Here's how the part is built. I have some questions about the finished solid (model axes, mm). A direction names the side the tool comes from. Give positions to 0.01 mm unless a question says otherwise; leave off trailing zeros. Loops run counter-clockwise (first coordinate to the right, second up) from the corner with the lowest first, then second, coordinate; pieces in that order, holes last. Notation, with made-up numbers: (58, 3) - (86, 3) arc R26 ccw to (86, 41) - close; hole circle Ø1 at (58, -14). An arc over 180 degrees is marked (long way). Use one line per item in the form item = value.
from build123d import *

# Parameters (mm, degrees)
SKETCH1_R           = 10
SKETCH1_R_2         = 5
BOSS_EXTRUDE1_DEPTH = 30
FILLET1_R           = 3


with BuildPart() as part:
    # Sketch1 → Boss-Extrude1 (new body)
    with BuildSketch(Plane.XY):
        Circle(SKETCH1_R)
        Circle(SKETCH1_R_2, mode=Mode.SUBTRACT)
    extrude(amount=BOSS_EXTRUDE1_DEPTH)

    # Sketch4 → Revolve1 (revolve)
    with BuildSketch(Plane(origin=(0, 0, 0), x_dir=(1, 0, 0), z_dir=(0, 1, 0))):
        Polygon((10, -5), (30, -5), (30, -7), (25, -9.886751346), (25, -20.113248654), (30, -23), (30, -25), (10, -25), align=None)
    revolve(axis=Axis((0, 0, 0), (0, 0, 1)))

    # Fillet1
    fillet1_edges = [part.edges().sort_by_distance(p)[0] for p in [
        (-25, 0, 20.113248654),
        (-25, 0, 9.886751346),
    ]]
    fillet(fillet1_edges, radius=FILLET1_R)


solid = part.part
(1) For P1, Ø6, axis at x = 0, y = 0, coming from the -Z side; P2, Ø12, axis at x = 9, y = -14, coming from the -Z side; P3, Ø1, axis at x = -12.5, z = 19.5, coming from the +Y side; P4, Ø3, axis at x = 10.5, z = 4.5, coming from the -Y side, each with a flat end and sliding along its axis, tell me the tip position at first contact or that it passes through.
Geometry says:
P1 = through
P2 = 5
P3 = 22.29
P4 = -28.59
(2) If I drill on probe 1 along Y at (x, z) = (0, 13.75); probe 2 along Z at (x, y) = (-14, -2.5); probe 3 along Z at (x, y) = (-25, 5), over which ranges is the centre line in solid material (lowest first)?
Geometry says:
probe_1 = -25 to -5, 5 to 25
probe_2 = 5 to 25
probe_3 = 5 to 9.97, 20.03 to 25
(3) If we section it at B-B (z = 12.5): List the corners of the cut face in (x, y) for me.
Geometry says:
outline = circle Ø50 at (0, 0); hole circle Ø10 at (0, 0)
(4) If we section it at A-A (z = 24.25): List the corners of the cut face in (x, y) for me.
Geometry says:
outline = circle Ø60 at (0, 0); hole circle Ø10 at (0, 0)
(5) Thinking about a two-plate mould opening in X: for faces 1 (the cylindrical face through (-3.255, 24.787, 15.047)), 2 (the cylindrical face through (-1.08, -4.88, 14.79)), 3 (the flat face through (-5, -2, 30)), which applies, pulls with the +X half, pulls with the -X half, needs draft (parallel to the pull), parting line crosses it, or undercut?
Geometry says:
face_1 = parting line crosses it
face_2 = undercut
face_3 = needs draft
(6) For faces 4 (the conical face through (25.49, 8.03, 21.11)), 5 (the flat face through (13, 0, 25)), 6 (the flat face through (-13, 0, 5)), which set-ups out of +Z, -Z, +X, -X, +Y, -Y let a thin tool reach every point of the face, with its end or its side?
Geometry says:
face_4 = none
face_5 = +Z
face_6 = -Z
